The model under review builds one solid part; all positions refer to its coordinate system, in mm. Face numbers are marked on the shaded views. A direction names the side the tool comes from. Round coordinates to 2 decimals unless told otherwise and drop trailing zeros. Loops run counter-clockwise (first coordinate to the right, second up) from the corner with the lowest first, then second, coordinate; pieces in that order, holes last. Notation, with made-up numbers: M 34,-17 L 39,-17 A30 cw 39,9 Z; hole C -5.5,-22 d11. An arc over 180 degrees is marked long. Answer in a Markdown table with one row per item. Add a question column.
from build123d import *

# Parameters (mm, degrees)
F2_R     = 4.25
F3_DEPTH = 13.9
F4_SIZE  = 0.5


with BuildPart() as f1:
    # F0 (on Front) → F1 (revolve)
    with BuildSketch(Plane.XZ):
        Polygon((0, 12.5), (0, 0), (13.9, 0), (13.9, 10.75), (9, 10.75), (9, 12.5), align=None)
    revolve(axis=Axis((6.95, 0, 0), (1, 0, 0)))

    # F2 (on face) → F3 (cut, through all)
    with BuildSketch(Plane(origin=(0, 0, 0), x_dir=(0, -1, 0), z_dir=(-1, 0, 0))):
        Circle(F2_R)
    extrude(amount=-F3_DEPTH, mode=Mode.SUBTRACT)

    # F4
    f4_edges = [f1.edges().sort_by_distance(p)[0] for p in [
        (13.9, 0, -10.75),
        (0, 0, -12.5),
    ]]
    chamfer(f4_edges, length=F4_SIZE)


solid = f1.part
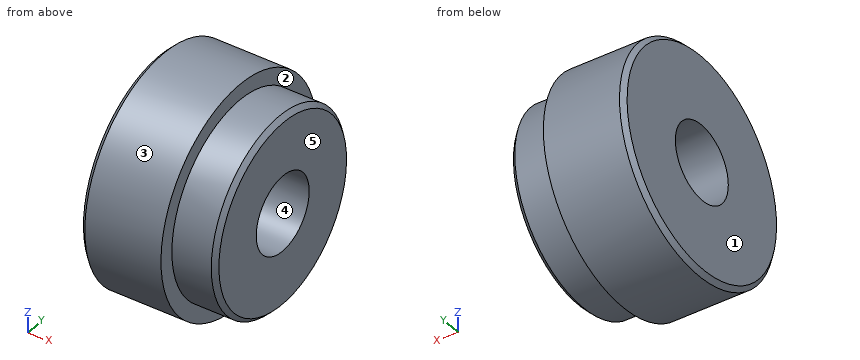
1. Take a section at A-A, the plane y = 0. State the section outline as (x, z) points, and give its area (3 significant figures).
2. For pin 1 Ø1.5 at (x, z) = (4, -8) entering from +Y; pin 2 Ø7 at (y, z) = (0, 0) entering from -X; pin 3 Ø1.5 at (x, z) = (9, -7) entering from +Y; pin 4 Ø1 at (x, y) = (2, -5) entering from -Z, all flat-tipped, find the tip position at first contact; note any pin that passes through.
3. Take a section at D-D, the plane x = 7.5. State the section outline as (y, z) points.
4. Mouldability with a two-part tool opening along Z and no side actions: class the marked faces 3, 4 and 5 as released by +Z, released by -Z, zero draft, split by the parting line, or undercut.
5. To check wall thickness, follow probe 1 along Z at (x, y) = (10.25, 0); probe 2 along Z at (x, y) = (2.5, 0); probe 3 along X at (y, z) = (10.75, 1). State the ranges of each line that lie inside material, in increasing order.
6. Machinability: for the marked faces 1 and 2, which of the approach directions +Z, -Z, +X, -X, +Y, -Y give a long, thin tool a straight path to every point of the face, cutting with its end or side? Answer none if there is none.
7. Take a section at C-C, the plane x = 12.25. State the section outline as (y, z) points, and give its area (3 significant figures).
Check sheet entries:
| question | item | result |
|---|---|---|
| 1 | outline | M 0,-12 L 0.5,-12.5 L 9,-12.5 L 9,-10.75 L 13.4,-10.75 L 13.9,-10.25 L 13.9,-4.25 L 0,-4.25 Z; M 0,4.25 L 13.9,4.25 L 13.9,10.25 L 13.4,10.75 L 9,10.75 L 9,12.5 L 0.5,12.5 L 0,12 Z |
| 1 | area | 212 mm^2 |
| 2 | pin 1 | stops at y = 10.18 |
| 2 | pin 2 | passes through |
| 2 | pin 3 | stops at y = 10.83 |
| 2 | pin 4 | stops at z = -11.66 |
| 3 | outline | C 0,0 d25; hole C 0,0 d8.5 |
| 4 | face 3 | split by the parting line |
| 4 | face 4 | undercut |
| 4 | face 5 | zero draft |
| 5 | probe 1 | z = -10.75 to -4.25, 4.25 to 10.75 |
| 5 | probe 2 | z = -12.5 to -4.25, 4.25 to 12.5 |
| 5 | probe 3 | x = 0 to 9 |
| 6 | face 1 | +Z, -Z, -X, +Y, -Y |
| 6 | face 2 | +X |
| 7 | outline | C 0,0 d21.5; hole C 0,0 d8.5 |
| 7 | area | 306 mm^2 |
